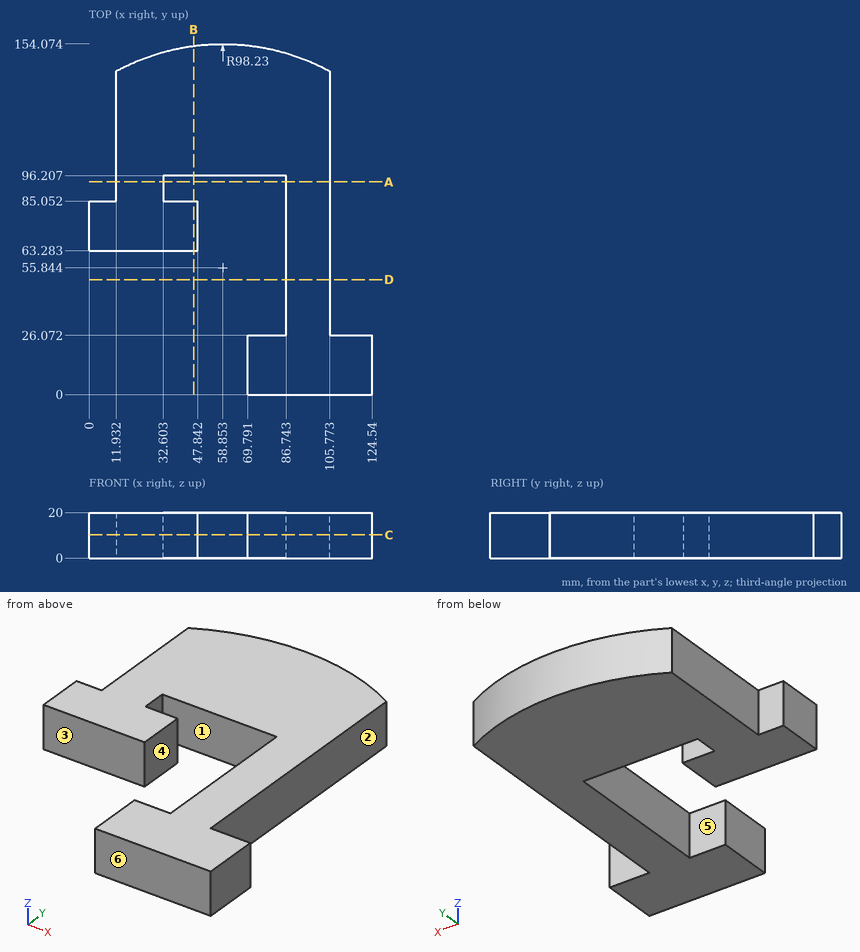
For this review, use the dimensioned drawing (mm, ordinates from the lowest corner) and the shaded views. A direction names the side the tool comes from. Give positions to 0.01 mm unless a question says otherwise; leave off trailing zeros. Order: outer loops, then holes, each group sorted by start corner. A loop starts at its lowest first (then second) coordinate and runs counter-clockwise, first axis right, second up. Notation, with made-up numbers: (84.25, 36) - (91.25, 36) arc R24 ccw to (91.25, 63) - close; hole circle Ø9 at (80, 15.25). An arc over 180 degrees is marked (long way). Use a Markdown table: item, result. Add a question column.
(1) Add section C-C on z = 10.25. Give the boundary of the cut face in (x, y).
(2) Add section A-A on y = 93.5. Give the boundary of the cut face in (x, z), then the cut area to 3 significant figures.
(3) Mouldability with a two-part tool opening along Y and no side actions: class the marked faces 4, 5 and 6 as +Y half, -Y half, draft (parallel to the pull), parting line (faces both ways), or undercut.
(4) Clearance check with flat-ended pins moving along their axes: P1, Ø4.5, axis at x = 36.5, z = 6, coming from the +Y side (1 decimal); P2, Ø4, axis at x = 75, z = 17.5, coming from the +Y side; P3, Ø5.5, axis at x = 113, z = 12.5, coming from the +Y side. State where each tip first meets the part, or that it passes through.
(5) Machinability: for the marked faces 1, 2 and 3, which of the approach directions +Z, -Z, +X, -X, +Y, -Y give a long, thin tool a straight path to every point of the face, cutting with its end or side? Answer none if there is none.
(6) Add section D-D on y = 50.5. Give the boundary of the cut face in (x, z).
(7) Add section B-B on x = 46. Give the boundary of the cut face in (y, z).
(8) Wall thickness on probe 1 along Y at (x, z) = (58, 19.25); probe 2 along X at (y, z) = (70, 4.75); probe 3 along X at (y, z) = (102.5, 7): over which ranges is each line inside the solid? List them lowest first. Write a range as [from, to].
Report:
| question | item | result |
|---|---|---|
| 1 | outline | (0, 63.28) - (47.84, 63.28) - (47.84, 85.05) - (32.6, 85.05) - (32.6, 96.21) - (86.74, 96.21) - (86.74, 26.07) - (69.79, 26.07) - (69.79, 0) - (124.54, 0) - (124.54, 26.07) - (105.77, 26.07) - (105.77, 142.14) arc R98.23 ccw to (11.93, 142.14) - (11.93, 85.05) - (0, 85.05) - close |
| 2 | outline | (11.93, 0) - (32.6, 0) - (32.6, 20) - (11.93, 20) - close; (86.74, 0) - (105.77, 0) - (105.77, 20) - (86.74, 20) - close |
| 2 | area | 794 mm² |
| 3 | face 4 | draft |
| 3 | face 5 | undercut |
| 3 | face 6 | -Y half |
| 4 | P1 | stops at y = 152 |
| 4 | P2 | stops at y = 153.05 |
| 4 | P3 | stops at y = 26.07 |
| 5 | face 1 | +Z, -Z |
| 5 | face 2 | +Z, -Z, +X, +Y |
| 5 | face 3 | +Z, -Z, -X, -Y |
| 6 | outline | (86.74, 0) - (105.77, 0) - (105.77, 20) - (86.74, 20) - close |
| 7 | outline | (63.28, 0) - (85.05, 0) - (85.05, 20) - (63.28, 20) - close; (96.21, 0) - (153.23, 0) - (153.23, 20) - (96.21, 20) - close |
| 8 | probe 1 | y = [96.21, 154.07] |
| 8 | probe 2 | x = [0, 47.84], [86.74, 105.77] |
| 8 | probe 3 | x = [11.93, 105.77] |
